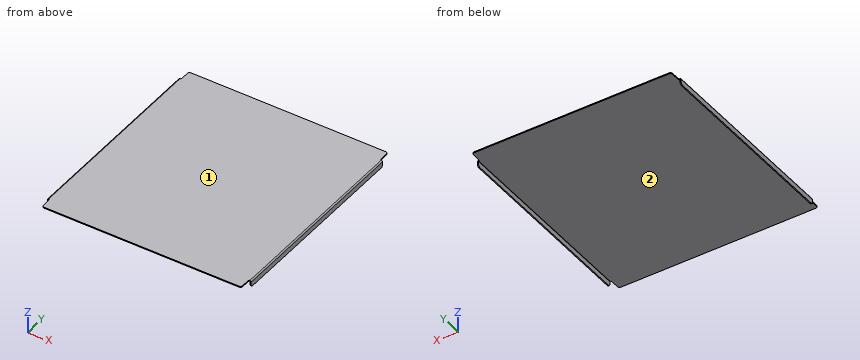
```python
from build123d import *

# Parameters (mm, degrees)
F0_W     = 938
F0_H     = 1040
F1_DEPTH = 5
F3_DEPTH = 465
F4_R     = 10
F5_R     = 5


# Not quite as in the source:
# - a pattern or mirror of a feature is missing from the dataset's text; its kind, count and spacing are read off the source's solid


with BuildPart() as f1:
    # F0 (on Top) → F1 (new body)
    with BuildSketch(Plane.XY):
        Rectangle(F0_W, F0_H)
    extrude(amount=F1_DEPTH)

    # F2 (on Front) → F3 (join, symmetric)
    with BuildSketch(Plane.XZ):
        with BuildLine():
            Line((-469, 0), (-469, 5))
            Line((-469, 5), (-474, 5))
            ThreePointArc((-474, 5), (-478.2426406871, 3.2426406871), (-480, -1))
            Line((-480, -1), (-480, -25))
            Line((-480, -25), (-475, -25))
            Line((-475, -25), (-475, -1))
            ThreePointArc((-475, -1), (-474.7071067812, -0.2928932188), (-474, 0))
            Line((-474, 0), (-469, 0))
        make_face()
    f3 = extrude(amount=F3_DEPTH, both=True)

    # F3_copies: F3 across plane
    add(f3.mirror(Plane(origin=(0, 0, 0), x_dir=(0, 0, 1), z_dir=(1, 0, 0))))

    # F4
    f4_edges = [f1.edges().sort_by_distance(p)[0] for p in [
        (-469, -520, 2.5),
        (-477.5, -465, -25),
        (-477.5, 465, -25),
        (-469, 520, 2.5),
        (469, 520, 2.5),
        (469, -520, 2.5),
        (477.5, -465, -25),
        (477.5, 465, -25),
    ]]
    fillet(f4_edges, radius=F4_R)

    # F5
    f5_edges = [f1.edges().sort_by_distance(p)[0] for p in [
        (-469, -465, 2.5),
        (-469, 465, 2.5),
        (469, -465, 2.5),
        (469, 465, 2.5),
    ]]
    fillet(f5_edges, radius=F5_R)


solid = f1.part
```
Work out the finished part from the listing and answer in its coordinate system (mm). Face numbers are marked on the shaded views. Give positions to 0.01 mm unless a question says otherwise; leave off trailing zeros. Loops run counter-clockwise (first coordinate to the right, second up) from the corner with the lowest first, then second, coordinate; pieces in that order, holes last. Notation, with made-up numbers: (-3.75, 6) - (31.25, 6) arc R12 ccw to (31.25, 23) - close; hole circle Ø8 at (61.5, 35.25). An arc over 180 degrees is marked (long way). One line per question, with ' | ' between items.
(1) The part is cut by section C-C (x = -190.5). Write down the section's boundary in (y, z).
Recorded:
outline: (-520, 0) - (520, 0) - (520, 5) - (-520, 5) - close
(2) Each of these flat-tipped pins is pushed along its axis until it touches: pin 1 Ø4 at (x, y) = (145.5, 38) entering from -Z; pin 2 Ø3 at (x, z) = (477, -1.5) entering from +Y; pin 3 Ø1.5 at (y, z) = (-496.5, 1.5) entering from +X; pin 4 Ø10 at (x, z) = (269.5, -9.5) entering from +Y. Where does it stop, or does it pass through?
Recorded:
pin 1: stops at z = 0 | pin 2: stops at y = 465 | pin 3: stops at x = 469 | pin 4: passes through
(3) The part is cut by section A-A (z = -10). Write down the section's boundary in (x, y).
Recorded:
outline: (-480, -465) - (-475, -465) - (-475, 465) - (-480, 465) - close; (475, -465) - (480, -465) - (480, 465) - (475, 465) - close
(4) The mould has two halves that part along X. Classify the marked faces 1 and 2: +X half, -X half, draft (parallel to the pull), parting line (faces both ways), or undercut.
Recorded:
face 1: draft | face 2: undercut
(5) Straight lines are drawn through the part: probe 1 along X at (y, z) = (-112, -17); probe 2 along Z at (x, y) = (366.5, -125); probe 3 along X at (y, z) = (-4, 2). For each, find the intervals that lie inside material, in ascending order.
Recorded:
probe 1: x = -480 to -475, 475 to 480 | probe 2: z = 0 to 5 | probe 3: x = -479.2 to 479.2
(6) The part is cut by section B-B (y = 139). Write down the section's boundary in (x, z), then the cut area to 3 significant figures.
Recorded:
outline: (-480, -25) - (-475, -25) - (-475, -1) arc R1 cw to (-474, 0) - (474, 0) arc R1 cw to (475, -1) - (475, -25) - (480, -25) - (480, -1) arc R6 ccw to (474, 5) - (-474, 5) arc R6 ccw to (-480, -1) - close | area: 5,030 mm²
